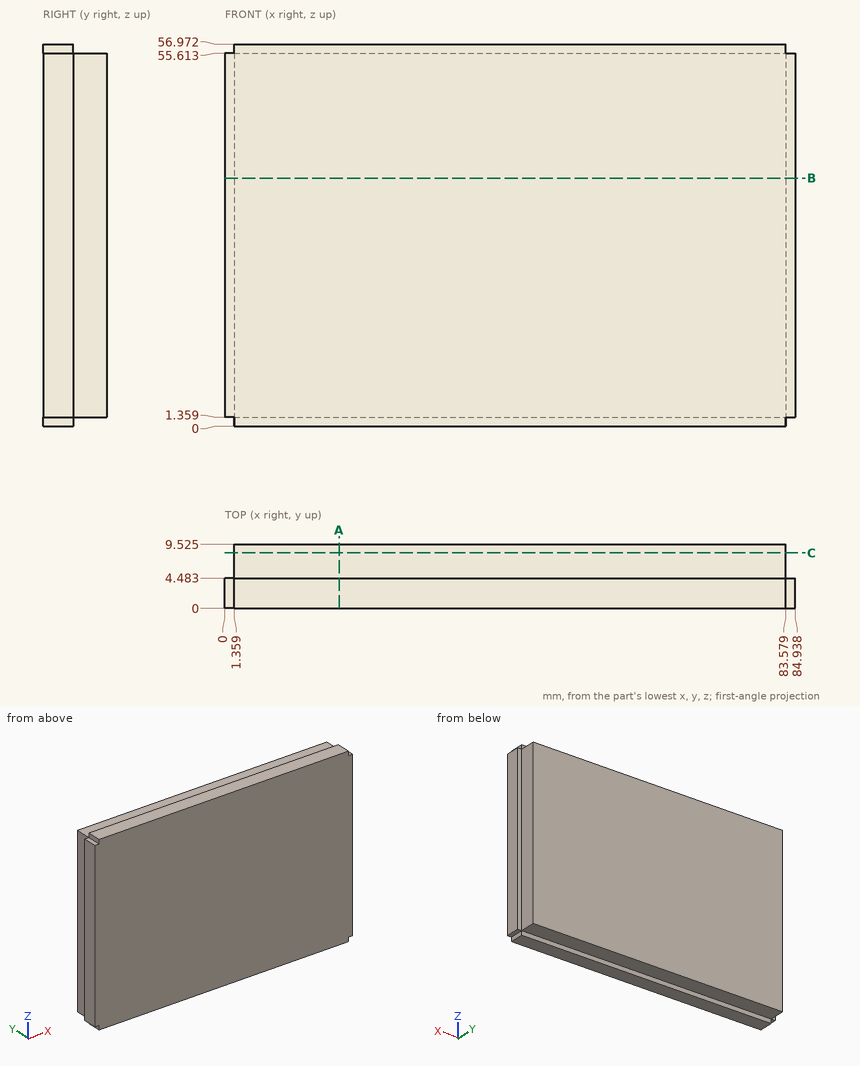
Study the drawing (mm; zero at the part's minimum x, y, z) and answer. Round coordinates to 2 decimals unless told otherwise and drop trailing zeros. Write each loop counter-clockwise with the first axis right and the second up, starting at its lowest first coordinate (ties: lowest second). Pieces come first, ordered by that corner, then holes. Notation, with made-up numbers: (64.25, 55.5) - (72.25, 55.5) arc R17 ccw to (72.25, 84.5) - close; hole circle Ø6 at (2, 72.5). An arc over 180 degrees is marked (long way). Return JSON: item names as keys, results as strings. Group by question number.
Q1. Find the intervals of material crossed by L1, parallel to X at y = 8, z = 38.5; L2, parallel to Z at x = 68, y = 7, in increasing order.
Q2. Each of these flat-tipped pins is pushed along its axis until it touches: pin 1 Ø2 at (y, z) = (7, 40) entering from -X; pin 2 Ø1.5 at (y, z) = (8, 20.5) entering from +X; pin 3 Ø0.7 at (x, y) = (0.5, 2.5) entering from -Z. Where does it stop, or does it pass through?
Q3. The part is cut by section C-C on y = 8.25. Write down the section's boundary in (x, z).
Q4. The part is cut by section A-A on x = 17. Write down the section's boundary in (y, z) (1 decimal), then the cut area to 3 significant figures.
Q5. The part is cut by section B-B on z = 37. Write down the section's boundary in (x, y) (1 decimal), then the cut area to 3 significant figures.
Solved:
{
 "1": {"L1": "1.36 to 83.58", "L2": "1.36 to 55.61"},
 "2": {"pin 1": "x = 1.36", "pin 2": "x = 83.58", "pin 3": "z = 1.36"},
 "3": {"outline": "(1.36, 1.36) - (83.58, 1.36) - (83.58, 55.61) - (1.36, 55.61) - close"},
 "4": {"outline": "(0, 0) - (4.5, 0) - (4.5, 1.4) - (9.5, 1.4) - (9.5, 55.6) - (4.5, 55.6) - (4.5, 57) - (0, 57) - close", "area": "529 mm²"},
 "5": {"outline": "(0, 0) - (84.9, 0) - (84.9, 4.5) - (83.6, 4.5) - (83.6, 9.5) - (1.4, 9.5) - (1.4, 4.5) - (0, 4.5) - close", "area": "795 mm²"}
}
